Can you work these out from the model? Positions are in its coordinate system, mm. Face numbers are marked on the shaded views. A direction names the side the tool comes from. Coordinates: 2 decimals unless noted, no trailing zeros. Order: outer loops, then holes, each group sorted by start corner. A loop starts at its lowest first (then second) coordinate and runs counter-clockwise, first axis right, second up. Notation, with made-up numbers: (11, 44) -> (55, 44) arc R17 cw to (55, 63) -> close; hole circle Ø11 at (-3.5, -17). An arc over 180 degrees is marked (long way). Write item = value, one per line.
```python
from build123d import *

# Parameters (mm, degrees)
SKETCH_W        = 52.4
SKETCH_H        = 52.4
PAD_DEPTH       = 6
SKETCH001_R     = 5.25
POCKET_DEPTH    = 5
SKETCH003_W     = 26.5
SKETCH003_H     = 9.486992
POCKET001_DEPTH = 24.5
PAD001_DEPTH    = 23.5


with BuildPart() as part:
    # Sketch → Pad (new body)
    with BuildSketch(Plane.XY):
        with Locations((26.2, -26.2)):
            Rectangle(SKETCH_W, SKETCH_H)
    extrude(amount=PAD_DEPTH)

    # Sketch001 (on Face6 of Pad) → Pocket (cut)
    with BuildSketch(Plane.XY.offset(6)):
        with Locations((6.5, -6.5)):
            Circle(SKETCH001_R)
        with Locations((45.9, -6.5)):
            Circle(SKETCH001_R)
        with Locations((45.9, -45.9)):
            Circle(SKETCH001_R)
        with Locations((6.5, -45.9)):
            Circle(SKETCH001_R)
    extrude(amount=-POCKET_DEPTH, mode=Mode.SUBTRACT)

    # Sketch003 (on DatumPlane) → Pocket001 (cut, symmetric)
    with BuildSketch(Plane.XZ.offset(26.2)):
        with Locations((26.2, 4.743496)):
            Rectangle(SKETCH003_W, SKETCH003_H)
    extrude(amount=POCKET001_DEPTH, both=True, mode=Mode.SUBTRACT)

    # Sketch004 (on DatumPlane) → Pad001 (join, symmetric)
    with BuildSketch(Plane.XZ.offset(26.2)):
        with BuildLine():
            ThreePointArc((25.45, 6.75), (20.2, 12), (14.95, 6.75))
            Line((14.95, 1.5), (14.95, 6.75))
            Line((12.95, 1.5), (14.95, 1.5))
            Line((12.95, 17), (12.95, 1.5))
            Line((12.95, 17), (39.45, 17))
            Line((39.45, 1.5), (39.45, 17))
            Line((37.45, 1.5), (39.45, 1.5))
            Line((37.45, 6.75), (37.45, 1.5))
            ThreePointArc((37.45, 6.75), (32.2, 12), (26.95, 6.75))
            Line((25.45, 6.75), (26.95, 6.75))
        make_face()
    extrude(amount=PAD001_DEPTH, both=True)


solid = part.part
```
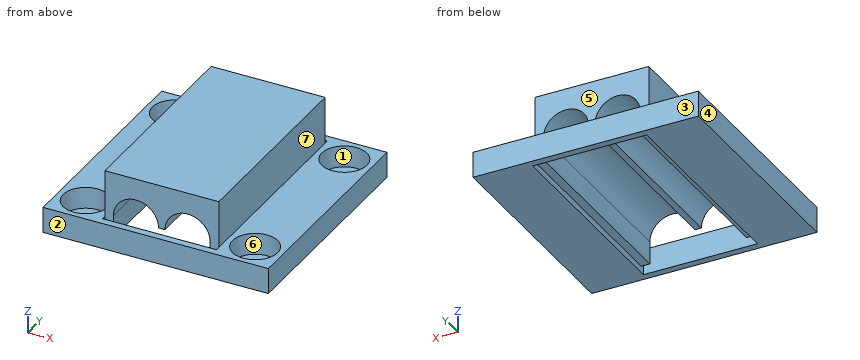
Item 1: I want a section at A-A, the plane x = 20.2. Please give me the cut outline in (y, z).
A:
outline = (-52.4, 0) -> (-50.7, 0) -> (-50.7, 6) -> (-52.4, 6) -> close; (-49.7, 12) -> (-2.7, 12) -> (-2.7, 17) -> (-49.7, 17) -> close; (-1.7, 0) -> (0, 0) -> (0, 6) -> (-1.7, 6) -> close
Item 2: If we mould it in two halves opening along Y, with no side actions, what happens to the marked faces 1, 2, 3 and 4? For each: pulls with the +Y half, pulls with the -Y half, needs draft (parallel to the pull), parting line crosses it, or undercut.
A:
face_1 = undercut
face_2 = pulls with the -Y half
face_3 = pulls with the +Y half
face_4 = needs draft
Item 3: I want a section at D-D, the plane z = 7.5. Please give me the cut outline in (x, y).
A:
outline = (12.95, -49.7) -> (15, -49.7) -> (15, -2.7) -> (12.95, -2.7) -> close; (25.4, -49.7) -> (27, -49.7) -> (27, -2.7) -> (25.4, -2.7) -> close; (37.4, -49.7) -> (39.45, -49.7) -> (39.45, -2.7) -> (37.4, -2.7) -> close
Item 4: I'm going to push flat-ended pins straight in: P1, Ø1.6, axis at x = 38.5, y = -28, coming from the -Z side; P2, Ø3.5, axis at y = -17, z = 11.5, coming from the +X side; P3, Ø12, axis at x = 6.5, y = -6.5, coming from the +Z side. Where does each tip first touch, or does it pass through?
A:
P1 = 1.5
P2 = 39.45
P3 = 6
Item 5: For the marked faces 5, 6 and 7, which set-ups out of +Z, -Z, +X, -X, +Y, -Y let a thin tool reach every point of the face, with its end or its side?
A:
face_5 = +Z, -Z
face_6 = +Z
face_7 = +Z, +X, +Y, -Y
Item 6: If I drill on probe 1 along Y at (x, z) = (45.9, 4.85); probe 2 along X at (y, z) = (-39.5, 3.5); probe 3 along X at (y, z) = (-16.5, 8.5), over which ranges is the centre line in solid material (lowest first)?
A:
probe_1 = -52.4 to -51.15, -40.65 to -11.75, -1.25 to 0
probe_2 = 0 to 14.95, 37.45 to 52.4
probe_3 = 12.95 to 15.25, 25.15 to 27.25, 37.15 to 39.45
Item 7: I want a section at B-B, the plane z = 4. Please give me the cut outline in (x, y).
A:
outline = (0, -52.4) -> (52.4, -52.4) -> (52.4, 0) -> (0, 0) -> close; hole circle Ø10.5 at (6.5, -45.9); hole circle Ø10.5 at (6.5, -6.5); hole (12.95, -50.7) -> (39.45, -50.7) -> (39.45, -49.7) -> (37.45, -49.7) -> (37.45, -2.7) -> (39.45, -2.7) -> (39.45, -1.7) -> (12.95, -1.7) -> (12.95, -2.7) -> (14.95, -2.7) -> (14.95, -49.7) -> (12.95, -49.7) -> close; hole circle Ø10.5 at (45.9, -45.9); hole circle Ø10.5 at (45.9, -6.5)
Item 8: I want a section at C-C, the plane y = -25.5. Please give me the cut outline in (x, z), plus the area to 3 significant figures.
A:
outline = (0, 0) -> (12.95, 0) -> (12.95, 1.5) -> (14.95, 1.5) -> (14.95, 6.75) arc R5.25 cw to (25.45, 6.75) -> (26.95, 6.75) arc R5.25 cw to (37.45, 6.75) -> (37.45, 1.5) -> (39.45, 1.5) -> (39.45, 0) -> (52.4, 0) -> (52.4, 6) -> (39.45, 6) -> (39.45, 17) -> (12.95, 17) -> (12.95, 6) -> (0, 6) -> close
area = 361 mm2
